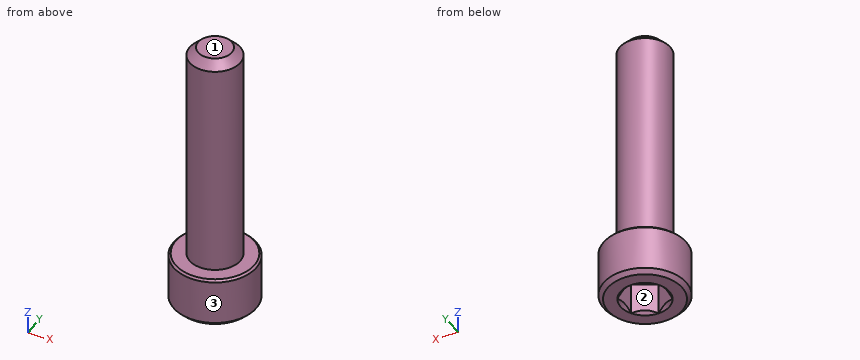
from build123d import *

# Parameters (mm, degrees)
SKETCH1_R          = 1.4224
EXTRUDE1_DEPTH     = 12.7
CHAMFER3_SIZE      = 0.47625
SKETCH6_R          = 2.3241
EXTRUDE2_DEPTH     = 2.8448
CUT_EXTRUDE1_DEPTH = 1.7859375
CHAMFER1_SIZE      = 0.23241
CHAMFER2_SIZE      = 0.116205


with BuildPart() as part:
    # Sketch1 → Extrude1 (new body)
    with BuildSketch(Plane.XY):
        Circle(SKETCH1_R)
    extrude(amount=-EXTRUDE1_DEPTH)

    # Chamfer3
    chamfer3_edges = [part.edges().sort_by_distance(p)[0] for p in [
        (-1.4224, 0, 0),
    ]]
    chamfer(chamfer3_edges, length=CHAMFER3_SIZE)

    # Sketch6 → Extrude2 (add)
    with BuildSketch(Plane(origin=(0, 0, -12.7), x_dir=(-1, 0, 0), z_dir=(0, 0, -1))):
        Circle(SKETCH6_R)
    extrude(amount=EXTRUDE2_DEPTH)

    # Sketch7 → Cut-Extrude1 (cut)
    with BuildSketch(Plane(origin=(0, 0, -15.5448), x_dir=(-1, 0, 0), z_dir=(0, 0, -1))):
        Polygon((0, 1.374815329), (-1.190625, 0.687407664), (-1.190625, -0.687407664), (0, -1.374815329), (1.190625, -0.687407664), (1.190625, 0.687407664), align=None)
    extrude(amount=-CUT_EXTRUDE1_DEPTH, mode=Mode.SUBTRACT)

    # Cut-Extrude2 cone 1 section (through the dimple's axis) → Cut-Extrude2 (revolve, cut)
    with BuildSketch(Plane(origin=(0, 0, -15.5448), x_dir=(0, 1, 0), z_dir=(1, 0, 0))):
        Polygon((0, 0), (1.374815329, 0), (0, 1.374815329), align=None)
    revolve(axis=Axis((0, 0, -15.5448), (0, 0, 1)), mode=Mode.SUBTRACT)

    # Chamfer1
    chamfer1_edges = [part.edges().sort_by_distance(p)[0] for p in [
        (2.3241, 0, -15.5448),
    ]]
    chamfer(chamfer1_edges, length=CHAMFER1_SIZE)

    # Chamfer2
    chamfer2_edges = [part.edges().sort_by_distance(p)[0] for p in [
        (2.3241, 0, -12.7),
    ]]
    chamfer(chamfer2_edges, length=CHAMFER2_SIZE)


solid = part.part
Work out the finished part from the listing and answer in its coordinate system (mm). Face numbers are marked on the shaded views. Round coordinates to 2 decimals unless told otherwise and drop trailing zeros. Write each loop counter-clockwise with the first axis right and the second up, starting at its lowest first coordinate (ties: lowest second). Pieces come first, ordered by that corner, then holes. Notation, with made-up numbers: M 40.25,7.25 L 79.25,7.25 A12 cw 79.25,25.25 Z; hole C 76.25,16.25 d11. An arc over 180 degrees is marked long. Use a Markdown table: item, result.
1) Flat-ended cylindrical pins translate along their axes: pin 1 (1 mm diameter, centred on y = 0, z = -10.5, fed in from -X); pin 2 (1.5 mm diameter, centred on y = -1.5, z = -10, fed in from +X). Find the tip coordinate at first contact, or state that the pin passes through.
Taken from the geometry:
| item | result |
|---|---|
| pin 1 | stops at x = -1.42 |
| pin 2 | stops at x = 1.21 |
2) The part is cut by section B-B on z = -6.75. Give the vertices of the cut face in (x, y), plus the area to 3 significant figures.
Taken from the geometry:
| item | result |
|---|---|
| outline | C 0,0 d2.84 |
| area | 6.36 mm2 |
3) Consider line 1 (Z direction, x = -0.8, y = -1.75); line 2 (Y direction, x = -0.1, z = -12.5); line 3 (X direction, y = 0.4, z = -14.5). Determine where each line is inside the solid, lowest interval first. Write a range as [from, to].
Taken from the geometry:
| item | result |
|---|---|
| line 1 | z = [-15.54, -12.7] |
| line 2 | y = [-1.42, 1.42] |
| line 3 | x = [-2.29, -1.19], [1.19, 2.29] |
4) The part is cut by section C-C on z = -13.5. Give the vertices of the cut face in (x, y).
Taken from the geometry:
| item | result |
|---|---|
| outline | C 0,0 d4.65 |
5) Determine the mould class of the marked faces 1, 2 and 3 for opening direction Y: pulls with the +Y half, pulls with the -Y half, needs draft (parallel to the pull), parting line crosses it, or undercut.
Taken from the geometry:
| item | result |
|---|---|
| face 1 | needs draft |
| face 2 | undercut |
| face 3 | parting line crosses it |
6) The part is cut by section A-A on y = 0. Give the vertices of the cut face in (x, z).
Taken from the geometry:
| item | result |
|---|---|
| outline | M -2.32,-15.31 L -2.09,-15.54 L -1.37,-15.54 L -1.19,-15.36 L -1.19,-13.76 L 1.19,-13.76 L 1.19,-15.36 L 1.37,-15.54 L 2.09,-15.54 L 2.32,-15.31 L 2.32,-12.82 L 2.21,-12.7 L 1.42,-12.7 L 1.42,-0.48 L 0.95,0 L -0.95,0 L -1.42,-0.48 L -1.42,-12.7 L -2.21,-12.7 L -2.32,-12.82 Z |
